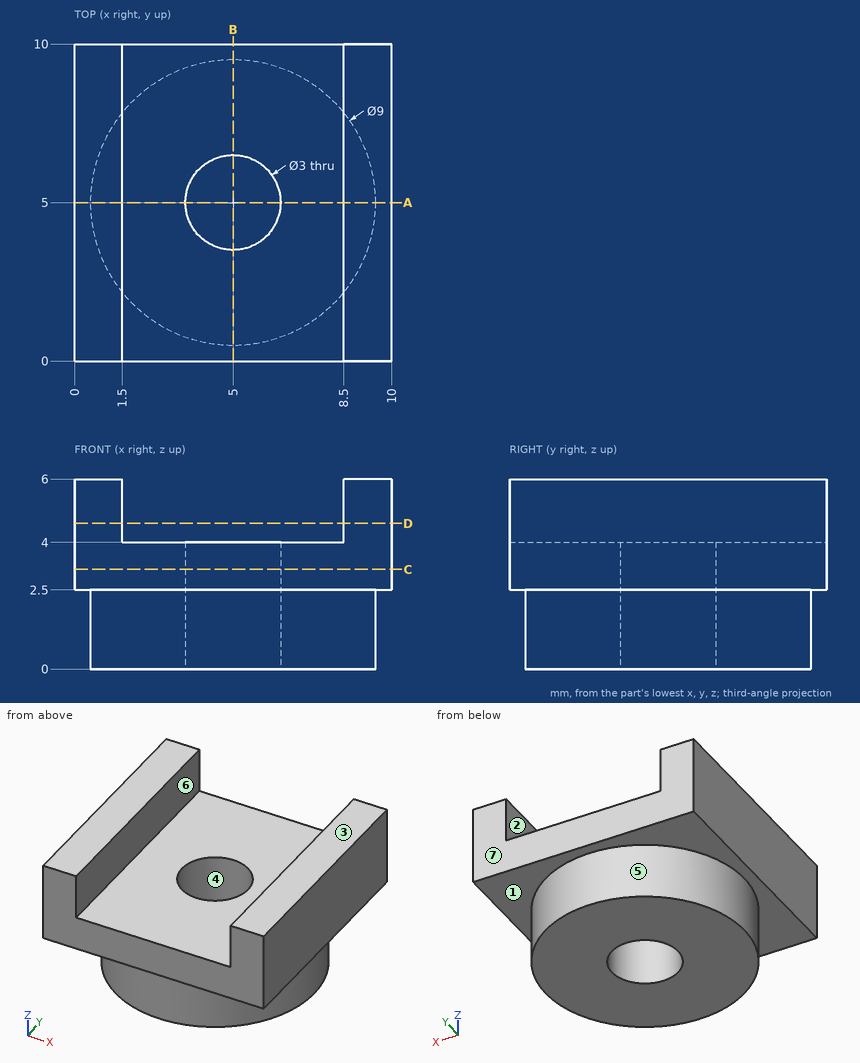
Job drawing, mm, ordinate dimensions from the low corner. One solid piece. A direction names the side the tool comes from. Round coordinates to 2 decimals unless told otherwise and drop trailing zeros. Loops run counter-clockwise (first coordinate to the right, second up) from the corner with the lowest first, then second, coordinate; pieces in that order, holes last.
(1) Cut at C-C (z = 3.15). Give the cut face in (x, y).
(2) Drop a flat-ended pin along its axis: pin 1 (5.5 mm diameter, centred on x = 6, y = 4, fed in from +Z). Give the stop position or say it passes through.
(3) Cut at A-A (y = 5). Give the cut face in (x, z), plus the area to 3 significant figures.
(4) Cut at D-D (z = 4.6). Give the cut face in (x, y), plus the area to 3 significant figures.
(5) Cut at B-B (x = 5). Give the cut face in (y, z).
(6) Wall check: line 1 along Y through (x, z) = (5, 1.6); line 2 along Z through (x, y) = (3, 0.75); line 3 along Z through (x, y) = (7.25, 3.75). Give the ranges that are in metal, low to high.
(7) Two-plate mould, pull along Y, no slides. Class the marked faces 4, 5, 6 and 7: +Y half, -Y half, draft (parallel to the pull), parting line (faces both ways), or undercut.
(8) Which spindle directions (+Z, -Z, +X, -X, +Y, -Y) get a long thin tool onto all of the face, cutting with end or side? Do the marked faces 1, 2 and 3. Say none if no direction does.
Findings below:
1. outline: (0, 0) - (10, 0) - (10, 10) - (0, 10) - close; hole circle Ø3 at (5, 5)
2. pin 1: stops at z = 6
3. outline: (0, 2.5) - (0.5, 2.5) - (0.5, 0) - (3.5, 0) - (3.5, 4) - (1.5, 4) - (1.5, 6) - (0, 6) - close; (6.5, 0) - (9.5, 0) - (9.5, 2.5) - (10, 2.5) - (10, 6) - (8.5, 6) - (8.5, 4) - (6.5, 4) - close
3. area: 31.5 mm2
4. outline: (0, 0) - (1.5, 0) - (1.5, 10) - (0, 10) - close; (8.5, 0) - (10, 0) - (10, 10) - (8.5, 10) - close
4. area: 30.0 mm2
5. outline: (0, 2.5) - (0.5, 2.5) - (0.5, 0) - (3.5, 0) - (3.5, 4) - (0, 4) - close; (6.5, 0) - (9.5, 0) - (9.5, 2.5) - (10, 2.5) - (10, 4) - (6.5, 4) - close
6. line 1: y = 0.5 to 3.5, 6.5 to 9.5
6. line 2: z = 2.5 to 4
6. line 3: z = 0 to 4
7. face 4: undercut
7. face 5: parting line
7. face 6: draft
7. face 7: +Y half
8. face 1: -Z
8. face 2: +Z, +Y, -Y
8. face 3: +Z, +X, -X, +Y, -Y
